Autodesk Inventor part; units mm, degrees
ref_plane "YZ Plane" through (0, 0, 0) normal (1, 0, 0) x (0, 1, 0)
ref_plane "XZ Plane" through (0, 0, 0) normal (0, 1, 0) x (-1, 0, 0)
ref_plane "XY Plane" through (0, 0, 0) normal (0, 0, 1) x (1, 0, 0)
sketch "Sketch1" plane through (0, 0, 0) normal (0, 0, 1) x (1, 0, 0)
  line L0 (0, 0) -> (30, 0)
  line L1 (30, 0) -> (30, 45)
  line L2 (30, 45) -> (0, 45)
  line L3 (0, 45) -> (0, 0)
  dimension "d0" = 30
  dimension "d1" = 45
extrude "Extrusion1" add sketch "Sketch1" along normal blind 40
sketch "Sketch2" plane through (0, 45, 0) normal (0, 1, 0) x (1, 0, 0)
  circle A0 centre (15, -17.7834) radius 7.5
  line L0 (30, -40) -> (0, -40)
  point P0 (0, 0)
  point P1 (15, -40)
  dimension "d4" = 15
  dimension "d5" = 22.2166
extrude "Extrusion2" cut sketch "Sketch2" against normal blind 5
sketch "Sketch3" plane through (30, 0, 0) normal (1, 0, 0) x (0, 0, -1)
  circle A0 centre (-31.5856, 6) radius 2.5
  line L0 (0, 0) -> (-40, 0)
  line L1 (-40, 0) -> (-40, 45)
  dimension "d8" = 5
  dimension "d9" = 6
  dimension "d10" = 8.4144
extrude "Extrusion3" cut sketch "Sketch3" against normal through all
sketch "Sketch4" plane through (0, 0, 40) normal (0, 0, 1) x (1, 0, 0)
  line L0 (0, 45) -> (0, 0)
  line L1 (30, 0) -> (30, 45)
  line L2 (0, 0) -> (30, 0)
  line L3 (1.5, 0) -> (28.5, 0)
  line L4 (28.5, 0) -> (28.5, 34.2)
  line L5 (28.5, 34.2) -> (1.5, 34.2)
  line L6 (1.5, 34.2) -> (1.5, 0)
  point P0 (15, 0)
  dimension "d13" = 27
  dimension "d14" = 34.2
extrude "Extrusion4" cut sketch "Sketch4" against normal through all
sketch "Sketch5" plane through (30, 0, 0) normal (1, 0, 0) x (0, 0, -1)
  line L0 (-24, 0) -> (0, 34.2)
  line L1 (0, 0) -> (0, 45)
  line L2 (0, 0) -> (-40, 0)
  point P0 (-40, 34.2)
  dimension "d17" = 24
extrude "Extrusion5" cut sketch "Sketch5" against normal through all
properties part number "link_b2" material "ABS Plastic"
The model under review builds one solid part; all positions refer to its coordinate system, in mm. A direction names the side the tool comes from. Coordinates: 2 decimals unless noted, no trailing zeros. Order: outer loops, then holes, each group sorted by start corner. A loop starts at its lowest first (then second) coordinate and runs counter-clockwise, first axis right, second up. Notation, with made-up numbers: (-27.5, 29.5) -> (-14.5, 29.5) arc R7 ccw to (-14.5, 33.5) -> close; hole circle Ø2 at (62, 4). An arc over 180 degrees is marked (long way). Answer in a Markdown table with one row per item. Add a question column.
Item 1: Machinability: for faces 1 (the flat face through (15, 40, 18)), 2 (the flat face through (29.26, 16.86, 12.17)), 3 (the flat face through (15, 34.2, 20)), which of the approach directions +Z, -Z, +X, -X, +Y, -Y give a long, thin tool a straight path to every point of the face, cutting with its end or side? Answer none if there is none.
Item 2: We need section B-B on x = 15. Write out the cut boundary in (y, z).
Item 3: Mouldability with a two-part tool opening along Z and no side actions: class faces 4 (the cylindrical face through (14.024, 42.535, 10.347)), 5 (the flat face through (0.76, 16.86, 12.17)), 6 (the cylindrical face through (29.26, 6.75, 29.2)), 7 (the flat face through (28.5, 21, 25)) as +Z half, -Z half, draft (parallel to the pull), parting line (faces both ways), or undercut.
Item 4: We need section A-A on z = 4. Write out the cut boundary in (x, y), plus the area to 3 significant figures.
Item 5: We need section D-D on y = 6. Write out the cut boundary in (x, z), plus the area to 3 significant figures.
Item 6: To check wall thickness, follow probe 1 along Z at (x, y) = (15, 42); probe 2 along X at (y, z) = (22, 11.5); probe 3 along Y at (x, z) = (26.5, 7). State the ranges of each line that lie inside material, in increasing order.
Item 7: Clearance check with flat-ended pins moving along their axes: pin 1 (6 mm diameter, centred on y = 6, z = 31.59, fed in from -X); pin 2 (8 mm diameter, centred on x = 19, z = 11.5, fed in from -Y). State where each tip first meets the part, or that it passes through.
Item 8: We need section C-C on y = 14.5. Write out the cut boundary in (x, z), plus the area to 3 significant figures.
Final values:
| question | item | result |
|---|---|---|
| 1 | face 1 | +Y |
| 1 | face 2 | -Z, +X, -X, -Y |
| 1 | face 3 | +Z, -Z, -Y |
| 2 | outline | (34.2, 0) -> (45, 0) -> (45, 10.28) -> (40, 10.28) -> (40, 25.28) -> (45, 25.28) -> (45, 40) -> (34.2, 40) -> close |
| 3 | face 4 | undercut |
| 3 | face 5 | -Z half |
| 3 | face 6 | undercut |
| 3 | face 7 | draft |
| 4 | outline | (0, 28.5) -> (1.5, 28.5) -> (1.5, 34.2) -> (28.5, 34.2) -> (28.5, 28.5) -> (30, 28.5) -> (30, 45) -> (0, 45) -> close |
| 4 | area | 341 mm2 |
| 5 | outline | (0, 19.79) -> (1.5, 19.79) -> (1.5, 29.09) -> (0, 29.09) -> close; (0, 34.09) -> (1.5, 34.09) -> (1.5, 40) -> (0, 40) -> close; (28.5, 19.79) -> (30, 19.79) -> (30, 29.09) -> (28.5, 29.09) -> close; (28.5, 34.09) -> (30, 34.09) -> (30, 40) -> (28.5, 40) -> close |
| 5 | area | 45.6 mm2 |
| 6 | probe 1 | z = 0 to 10.28, 25.28 to 40 |
| 6 | probe 2 | x = 0 to 1.5, 28.5 to 30 |
| 6 | probe 3 | y = 34.2 to 45 |
| 7 | pin 1 | stops at x = 0 |
| 7 | pin 2 | stops at y = 34.2 |
| 8 | outline | (0, 13.82) -> (1.5, 13.82) -> (1.5, 40) -> (0, 40) -> close; (28.5, 13.82) -> (30, 13.82) -> (30, 40) -> (28.5, 40) -> close |
| 8 | area | 78.5 mm2 |
